Design review of the part shown in the three views and the two pictorial views. Dimensions are in mm from the part's minimum x, y and z. A direction names the side the tool comes from. Coordinates: 2 decimals unless noted, no trailing zeros. Loops run counter-clockwise (first coordinate to the right, second up) from the corner with the lowest first, then second, coordinate; pieces in that order, holes last. Notation, with made-up numbers: (9, 45) -> (34, 45) arc R32 cw to (34, 80) -> close; hole circle Ø2 at (-1.5, -17). An arc over 180 degrees is marked (long way). Answer in a Markdown table with one row per item.
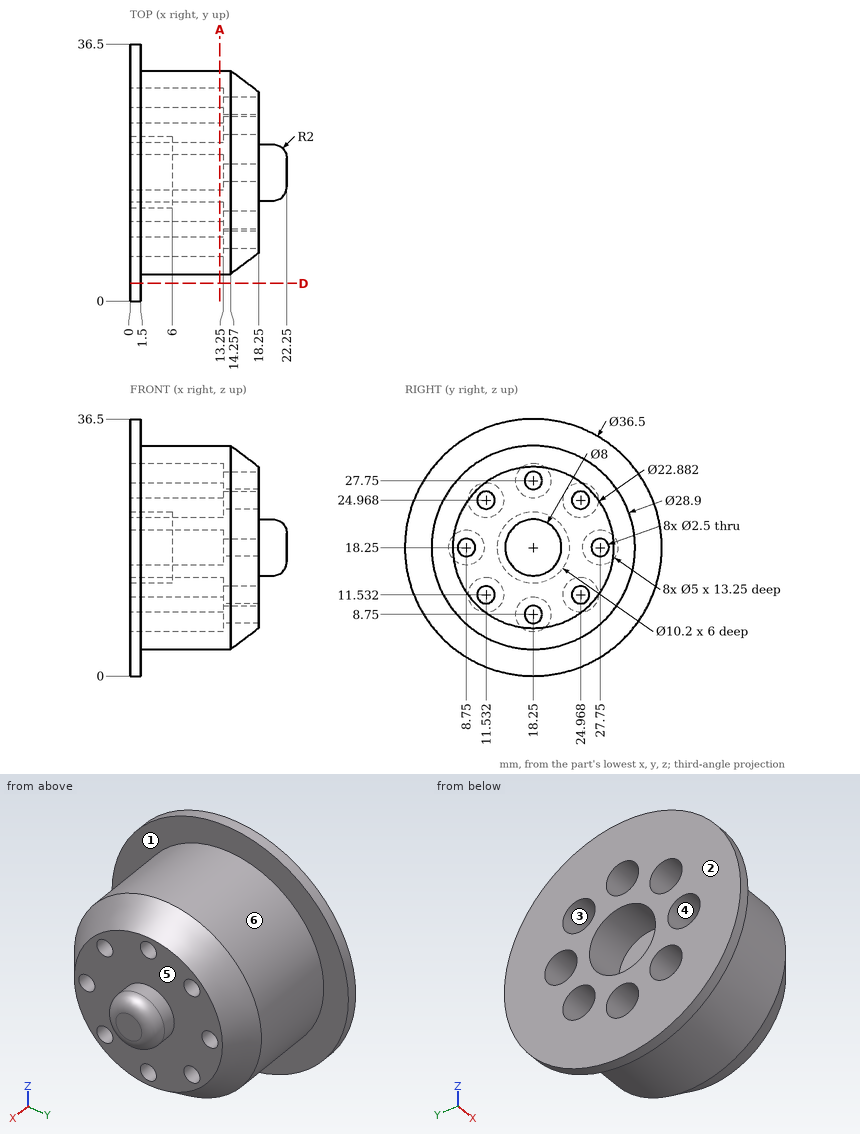
Item 1: For the marked faces 1, 2 and 3, list the 3-axis set-ups (+Z, -Z, +X, -X, +Y, -Y) from which the entire face can be reached by the end or side of a thin tool; tool diameter is ignored.
Worked answers:
| item | result |
|---|---|
| face 1 | +X |
| face 2 | +Z, -Z, -X, +Y, -Y |
| face 3 | -X |
Item 2: Take a section at A-A, the plane x = 12.75. Count the separate pieces of the cut face and the enclosed holes in it, and give its area (3 significant figures).
Worked answers:
| item | result |
|---|---|
| separate pieces | 1 |
| enclosed holes | 8 |
| area | 499 mm² |
Item 3: Insertion check: pin 1 (3 mm diameter, centred on y = 18.25, z = 8.75, fed in from -X); pin 2 (1.5 mm diameter, centred on y = 21.5, z = 9.5, fed in from +X); pin 3 (6 mm diameter, centred on x = 7.5, z = 9, fed in from -Y). Each pin has a flat end and moves straight along its axis. Give the tip position at first contact, or say it passes through.
Worked answers:
| item | result |
|---|---|
| pin 1 | x = 13.25 |
| pin 2 | x = 18.25 |
| pin 3 | y = 5.22 |
Item 4: For L1, parallel to Z at x = 10.25, y = 23.5 (1 decimal); L2, parallel to Y at x = 6.5, z = 10.5 (1 decimal); L3, parallel to Y at x = 8.75, z = 11.5 (1 decimal), list the stretches that pass through material, from the lowest coordinate up.
Worked answers:
| item | result |
|---|---|
| L1 | 4.8 to 9.5, 13.6 to 22.9, 27 to 31.7 |
| L2 | 6.1 to 9.3, 13.8 to 16.5, 20 to 22.7, 27.2 to 30.4 |
| L3 | 5.5 to 9, 14 to 22.5, 27.5 to 31 |
Item 5: The part is to be moulded in two halves that separate along Z. For the marked faces 4, 5 and 6, say which applies: +Z half, -Z half, draft (parallel to the pull), parting line (faces both ways), or undercut.
Worked answers:
| item | result |
|---|---|
| face 4 | undercut |
| face 5 | draft |
| face 6 | parting line |
Item 6: Take a section at D-D, the plane y = 2.5. State the section outline as (x, z) points.
Worked answers:
| item | result |
|---|---|
| outline | (0, 9.03) -> (1.5, 9.03) -> (1.5, 27.47) -> (0, 27.47) -> close |
